from build123d import *

# Parameters (mm, degrees)
SKETCH1_W               = 100
SKETCH1_H               = 76
SKETCH1_W_2             = 94
SKETCH1_H_2             = 70
BOSS_EXTRUDE1_DEPTH     = 389.5
CUT_EXTRUDE1_DEPTH      = 395.530417078
CUT_EXTRUDE1_DEPTH_BACK = 395.530417078
SKETCH4_W               = 64
SKETCH4_H               = 60
FILLET1_R               = 2


with BuildPart() as part:
    # Sketch1 → Boss-Extrude1 (new body)
    with BuildSketch(Plane(origin=(0, 0, 0), x_dir=(1, 0, 0), z_dir=(0, 1, 0))):
        Rectangle(SKETCH1_W, SKETCH1_H)
        Rectangle(SKETCH1_W_2, SKETCH1_H_2, mode=Mode.SUBTRACT)
    extrude(amount=BOSS_EXTRUDE1_DEPTH)

    # Sketch4 → Cut-Extrude1 (cut, two sides: drawn at the far end of the back side and taken through both)
    with BuildSketch(Plane(origin=(0, 0, 0), x_dir=(0, 0, -1), z_dir=(1, 0, 0)).offset(-CUT_EXTRUDE1_DEPTH_BACK)):
        with Locations((0, 30)):
            Rectangle(SKETCH4_W, SKETCH4_H)
    extrude(amount=CUT_EXTRUDE1_DEPTH + CUT_EXTRUDE1_DEPTH_BACK, mode=Mode.SUBTRACT)

    # Fillet1
    # the kernel refuses this fillet: 2 mm, written as the material it adds along each edge
    with BuildSketch(Plane(origin=(47, 0, 35), x_dir=(0, 0, -1), z_dir=(0, 1, 0))) as fillet1_piece_1:
        with BuildLine():
            CenterArc((FILLET1_R, FILLET1_R), FILLET1_R, 180, 90)
            Line((0, FILLET1_R), (0, 0))
            Line((0, 0), (FILLET1_R, 0))
        make_face()
    extrude(amount=389.5)
    with BuildSketch(Plane(origin=(-47, 0, 35), x_dir=(0, 0, -1), z_dir=(0, 1, 0)), Plane(origin=(47, 0, -35), x_dir=(0, 0, 1), z_dir=(0, 1, 0)), Plane(origin=(-47, 0, -35), x_dir=(1, 0, 0), z_dir=(0, 1, 0))) as fillet1_piece_2:
        with BuildLine():
            CenterArc((FILLET1_R, -FILLET1_R), FILLET1_R, 90, 90)
            Line((0, -FILLET1_R), (0, 0))
            Line((0, 0), (FILLET1_R, 0))
        make_face()
    extrude(amount=389.5)
    # the kernel refuses this fillet: 2 mm, written as the material it takes off along each edge
    with BuildSketch(Plane(origin=(50, -5, -38), x_dir=(-1, 0, 0), z_dir=(0, 1, 0)), Plane(origin=(-50, -5, -38), x_dir=(0, 0, 1), z_dir=(0, 1, 0))) as fillet1_2_piece_1:
        with BuildLine():
            CenterArc((FILLET1_R, FILLET1_R), FILLET1_R, 180, 90)
            Line((0, FILLET1_R), (0, 0))
            Line((0, 0), (FILLET1_R, 0))
        make_face()
    extrude(amount=399.5, mode=Mode.SUBTRACT)
    with BuildSketch(Plane(origin=(-50, -5, 38), x_dir=(0, 0, -1), z_dir=(0, 1, 0)), Plane(origin=(50, -5, 38), x_dir=(-1, 0, 0), z_dir=(0, 1, 0))) as fillet1_2_piece_2:
        with BuildLine():
            CenterArc((FILLET1_R, -FILLET1_R), FILLET1_R, 90, 90)
            Line((0, -FILLET1_R), (0, 0))
            Line((0, 0), (FILLET1_R, 0))
        make_face()
    extrude(amount=399.5, mode=Mode.SUBTRACT)
    with BuildSketch(Plane(origin=(-50, 60, 32), x_dir=(0, 1, 0), z_dir=(0, 0, -1)), Plane(origin=(50, 60, -32), x_dir=(0, 1, 0), z_dir=(0, 0, 1)), Plane(origin=(47, 60, 32), x_dir=(0, 1, 0), z_dir=(0, 0, -1))) as fillet1_2_piece_3:
        with BuildLine():
            CenterArc((FILLET1_R, FILLET1_R), FILLET1_R, 180, 90)
            Line((0, FILLET1_R), (0, 0))
            Line((0, 0), (FILLET1_R, 0))
        make_face()
    extrude(amount=64, mode=Mode.SUBTRACT)
    with BuildSketch(Plane(origin=(-47, 60, -32), x_dir=(-1, 0, 0), z_dir=(0, 0, 1))) as fillet1_2_piece_4:
        with BuildLine():
            CenterArc((FILLET1_R, -FILLET1_R), FILLET1_R, 90, 90)
            Line((0, -FILLET1_R), (0, 0))
            Line((0, 0), (FILLET1_R, 0))
        make_face()
    extrude(amount=64, mode=Mode.SUBTRACT)


solid = part.part
Could you check a few things on this model? Use its own coordinates, in mm. A direction names the side the tool comes from. Give positions to 0.01 mm unless a question says otherwise; leave off trailing zeros. Write each loop counter-clockwise with the first axis right and the second up, starting at its lowest first coordinate (ties: lowest second). Pieces come first, ordered by that corner, then holes. Notation, with made-up numbers: (5.25, 49) -> (51.25, 49) arc R18 cw to (51.25, 65) -> close; hole circle Ø11 at (62.5, 65.5). An arc over 180 degrees is marked (long way). Write each question's results on one line, items separated by ' | '. Start each with the question number.
Q1. Which directions (+Z, -Z, +X, -X, +Y, -Y) give clear straight access to the entire face, cutting with the end or side of a thin tool? Please do faces 5 (the face through (-1, 192, 38)), 6 (the face through (-1, 192, 35)).
Q2. Suppose I cut it at C-C, the plane y = 29. List the corners of the cut face in (x, z) for me.
Q3. Suppose I cut it at B-B, the plane z = 14. List the corners of the cut face in (x, y) for me, and give its area (3 significant figures).
Q4. We'd pull the mould along Z, two halves only. Please class faces 1 (the face through (-47, 235, 0)), 2 (the face through (0, 389.5, -37)), 3 (the face through (-1, 192, -35)), 4 (the face through (-1, 192, -38)): +Z half, -Z half, draft (parallel to the pull), parting line (faces both ways), or undercut.
Q5. Suppose I cut it at A-A, the plane x = 25. List the corners of the cut face in (y, z) for me, and give its area (3 significant figures).
Q6. I need wall thicknesses on probe 1 along Z at (x, y) = (30.5, 74.5); probe 2 along X at (y, z) = (86.5, -6). Which ranges of each line are inside material? Lowest first, please.
Q7. Suppose I cut it at D-D, the plane y = 224. List the corners of the cut face in (x, z) for me.
Outcome:
1) face 5: +Z, +X, -X, +Y, -Y | face 6: +Y, -Y
2) outline: (-50, -36) arc R2 ccw to (-48, -38) -> (48, -38) arc R2 ccw to (50, -36) -> (50, -32) -> (47, -32) -> (47, -33) arc R2 cw to (45, -35) -> (-45, -35) arc R2 cw to (-47, -33) -> (-47, -32) -> (-50, -32) -> close; (-50, 32) -> (-47, 32) -> (-47, 33) arc R2 cw to (-45, 35) -> (45, 35) arc R2 cw to (47, 33) -> (47, 32) -> (50, 32) -> (50, 36) arc R2 ccw to (48, 38) -> (-48, 38) arc R2 ccw to (-50, 36) -> close
3) outline: (-50, 62) arc R2 ccw to (-48.5, 60.06) arc R2 ccw to (-47, 62) -> (-47, 389.5) -> (-50, 389.5) -> close; (47, 62) arc R2 ccw to (48.5, 60.06) arc R2 ccw to (50, 62) -> (50, 389.5) -> (47, 389.5) -> close | area: 1,970 mm2
4) face 1: undercut | face 2: draft | face 3: undercut | face 4: -Z half
5) outline: (0, -38) -> (389.5, -38) -> (389.5, -35) -> (0, -35) -> close; (0, 35) -> (389.5, 35) -> (389.5, 38) -> (0, 38) -> close | area: 2,340 mm2
6) probe 1: -38 to -35, 35 to 38 | probe 2: -50 to -47, 47 to 50
7) outline: (-50, -36) arc R2 ccw to (-48, -38) -> (48, -38) arc R2 ccw to (50, -36) -> (50, 36) arc R2 ccw to (48, 38) -> (-48, 38) arc R2 ccw to (-50, 36) -> close; hole (-47, -33) arc R2 ccw to (-45, -35) -> (45, -35) arc R2 ccw to (47, -33) -> (47, 33) arc R2 ccw to (45, 35) -> (-45, 35) arc R2 ccw to (-47, 33) -> close
